Design review of the part built by this model. Coordinates are the model's own, in mm. A direction names the side the tool comes from. Coordinates: 2 decimals unless noted, no trailing zeros. Write each loop counter-clockwise with the first axis right and the second up, starting at its lowest first coordinate (ties: lowest second). Pieces come first, ordered by that corner, then holes. Notation, with made-up numbers: (66.25, -12.75) - (91.25, -12.75) arc R17 ccw to (91.25, -1.75) - close; hole circle Ø11 at (-34, 80.25). An arc over 180 degrees is marked (long way). Use a Markdown table: item, result.
from build123d import *

# Parameters (mm, degrees)
ESBO_O1_W                 = 50
ESBO_O1_H                 = 11
RESSALTO_EXTRUS_O1_DEPTH  = 22.5
ESBO_O2_W                 = 46
ESBO_O2_H                 = 7
CORTE_EXTRUS_O1_DEPTH     = 20.5
ESBO_O3_W                 = 10.97916057
ESBO_O3_H                 = 2
CORTE_EXTRUS_O2_DEPTH     = 4
CORTE_EXTRUS_O3_DEPTH     = 4
ESBO_O9_W                 = 50
ESBO_O9_H                 = 4
RESSALTO_EXTRUS_O4_DEPTH  = 7
ESBO_O13_R                = 1.5
CORTE_EXTRUS_O4_DEPTH     = 7
ESBO_O19_W                = 9
ESBO_O19_H                = 4
RESSALTO_EXTRUS_O5_DEPTH  = 22.5
ESBO_O20_W                = 50
ESBO_O20_H                = 4
CORTE_EXTRUS_O5_DEPTH     = 7
RESSALTO_EXTRUS_O6_DEPTH  = 0.75
RESSALTO_EXTRUS_O7_DEPTH  = 1.2
RESSALTO_EXTRUS_O8_DEPTH  = 1.5
RESSALTO_EXTRUS_O9_DEPTH  = 4.5
ESBO_O26_R                = 2.9
CORTE_EXTRUS_O6_DEPTH     = 4
ESBO_O28_W                = 7
ESBO_O28_H                = 7
RESSALTO_EXTRUS_O10_DEPTH = 4.5
CHANFRO1_SIZE             = 5
CHANFRO1_SIZE_2           = 3.372542584
CHANFRO2_SIZE             = 3.372542584
CHANFRO2_SIZE_2           = 5
CHANFRO3_SIZE             = 5
CHANFRO3_SIZE2            = 0.881634904
CHANFRO4_SIZE             = 5
CHANFRO4_SIZE2            = 1.919320175


with BuildPart() as part:
    # Esboço1 → Ressalto-extrusão1 (new body)
    with BuildSketch(Plane(origin=(0, 0, 0), x_dir=(1, 0, 0), z_dir=(0, 1, 0))):
        Rectangle(ESBO_O1_W, ESBO_O1_H)
    extrude(amount=RESSALTO_EXTRUS_O1_DEPTH)

    # Esboço2 → Corte-extrusão1 (cut)
    with BuildSketch(Plane(origin=(0, 22.5, 0), x_dir=(1, 0, 0), z_dir=(0, 1, 0))):
        Rectangle(ESBO_O2_W, ESBO_O2_H)
    extrude(amount=-CORTE_EXTRUS_O1_DEPTH, mode=Mode.SUBTRACT)

    # Esboço3 → Corte-extrusão2 (cut)
    with BuildSketch(Plane(origin=(0, 22.5, 0), x_dir=(1, 0, 0), z_dir=(0, 1, 0))):
        with Locations((0, 4.5)):
            Rectangle(ESBO_O3_W, ESBO_O3_H)
    extrude(amount=-CORTE_EXTRUS_O2_DEPTH, mode=Mode.SUBTRACT)

    # Esboço5 → Corte-extrusão3 (cut)
    with BuildSketch(Plane.XY.offset(5.5)):
        with BuildLine():
            Line((-21, 22.5), (-4.5, 22.5))
            Line((-4.5, 22.5), (-4.5, 11.75))
            ThreePointArc((-4.5, 11.75), (-12.75, 3.5), (-21, 11.75))
            Line((-21, 11.75), (-21, 22.5))
        make_face()
        with BuildLine():
            Line((4.5, 22.5), (21, 22.5))
            Line((21, 22.5), (21, 11.75))
            ThreePointArc((21, 11.75), (12.75, 3.5), (4.5, 11.75))
            Line((4.5, 11.75), (4.5, 22.5))
        make_face()
    extrude(amount=-CORTE_EXTRUS_O3_DEPTH, mode=Mode.SUBTRACT)

    # Esboço9 → Ressalto-extrusão4 (add)
    with BuildSketch(Plane(origin=(0, 0, -5.5), x_dir=(-1, 0, 0), z_dir=(0, 0, -1))):
        with Locations((0, 2)):
            Rectangle(ESBO_O9_W, ESBO_O9_H)
    extrude(amount=RESSALTO_EXTRUS_O4_DEPTH)

    # Esboço13 → Corte-extrusão4 (cut)
    with BuildSketch(Plane(origin=(0, 4, 0), x_dir=(1, 0, 0), z_dir=(0, 1, 0))):
        with Locations(Location((10, 9, 0), (0, 0, 270))):
            Circle(ESBO_O13_R)
        with Locations(Location((5, 9, 0), (0, 0, 270))):
            Circle(ESBO_O13_R)
        with Locations(Location((20, 9, 0), (0, 0, 270))):
            Circle(ESBO_O13_R)
        with Locations(Location((15, 9, 0), (0, 0, 270))):
            Circle(ESBO_O13_R)
        with Locations(Location((0, 9, 0), (0, 0, 270))):
            Circle(ESBO_O13_R)
        with Locations(Location((-5, 9, 0), (0, 0, 270))):
            Circle(ESBO_O13_R)
        with Locations(Location((-10, 9, 0), (0, 0, 270))):
            Circle(ESBO_O13_R)
        with Locations(Location((-15, 9, 0), (0, 0, 270))):
            Circle(ESBO_O13_R)
        with Locations(Location((-20, 9, 0), (0, 0, 270))):
            Circle(ESBO_O13_R)
    extrude(amount=-CORTE_EXTRUS_O4_DEPTH, mode=Mode.SUBTRACT)

    # Esboço19 → Ressalto-extrusão5 (add)
    with BuildSketch(Plane(origin=(0, 22.5, 0), x_dir=(1, 0, 0), z_dir=(0, 1, 0))):
        with Locations((0, -5.5)):
            Rectangle(ESBO_O19_W, ESBO_O19_H)
    extrude(amount=-RESSALTO_EXTRUS_O5_DEPTH)

    # Esboço20 → Corte-extrusão5 (cut)
    with BuildSketch(Plane(origin=(0, 0, -12.5), x_dir=(-1, 0, 0), z_dir=(0, 0, -1))):
        with Locations((0, 2)):
            Rectangle(ESBO_O20_W, ESBO_O20_H)
    extrude(amount=-CORTE_EXTRUS_O5_DEPTH, mode=Mode.SUBTRACT)

    # Esboço21 → Ressalto-extrusão6 (add)
    with BuildSketch(Plane(origin=(0, 22.5, 0), x_dir=(1, 0, 0), z_dir=(0, 1, 0))):
        Polygon((-21, -5.5), (-21, -3.5), (-23, -3.5), (-23, 3.5), (-5.489580285, 3.5), (-5.489580285, 5.5), (-25, 5.5), (-25, -5.5), align=None)
        Polygon((21, -3.5), (21, -5.5), (25, -5.5), (25, 5.5), (5.489580285, 5.5), (5.489580285, 3.5), (23, 3.5), (23, -3.5), align=None)
    extrude(amount=RESSALTO_EXTRUS_O6_DEPTH)

    # Esboço22 → Ressalto-extrusão7 (add)
    with BuildSketch(Plane(origin=(0, 23.25, 0), x_dir=(1, 0, 0), z_dir=(0, 1, 0))):
        Polygon((-24, 3.5), (-24, -5.5), (-25, -5.5), (-25, 5.5), (-5.489580285, 5.5), (-5.489580285, 4.5), (-23, 4.5), (-24, 4.5), align=None)
        Polygon((23, 4.5), (5.489580285, 4.5), (5.489580285, 5.5), (25, 5.5), (25, -5.5), (24, -5.5), (24, 3.5), (24, 4.5), align=None)
    extrude(amount=RESSALTO_EXTRUS_O7_DEPTH)

    # Esboço23 → Ressalto-extrusão8 (add)
    with BuildSketch(Plane(origin=(0, 24.45, 0), x_dir=(1, 0, 0), z_dir=(0, 1, 0))):
        Polygon((-24, 4.5), (-24, -5.5), (-25, -5.5), (-25, 5.5), (-5.489580285, 5.5), (-5.489580285, 4.5), align=None)
        Polygon((-23, 3.5), (-5.489580285, 3.5), (-5.489580285, 4.5), (-24, 4.5), (-24, -5.5), (-21, -5.5), (-21, -3.5), (-23, -3.5), align=None)
        Polygon((5.489580285, 5.5), (5.489580285, 4.5), (24, 4.5), (24, -5.5), (25, -5.5), (25, 5.5), align=None)
        Polygon((23, -3.5), (21, -3.5), (21, -5.5), (24, -5.5), (24, 4.5), (5.489580285, 4.5), (5.489580285, 3.5), (23, 3.5), align=None)
    extrude(amount=RESSALTO_EXTRUS_O8_DEPTH)

    # Esboço24 → Ressalto-extrusão9 (add)
    with BuildSketch(Plane.XZ):
        Polygon((0, 3.5), (-3.5, 3.5), (-3.5, 0), (-3.5, -3.5), (3.5, -3.5), (3.5, 3.5), align=None)
    extrude(amount=RESSALTO_EXTRUS_O9_DEPTH)

    # Esboço26 → Corte-extrusão6 (cut)
    with BuildSketch(Plane.XZ.offset(4.5)):
        with Locations(Location((0, 0, 0), (0, 0, 270))):
            Circle(ESBO_O26_R)
    extrude(amount=-CORTE_EXTRUS_O6_DEPTH, mode=Mode.SUBTRACT)

    # Esboço28 → Ressalto-extrusão10 (add)
    with BuildSketch(Plane.XZ):
        Polygon((-4.5, 5.5), (-9.5, 5.5), (-9.5, -5.5), (9.5, -5.5), (9.5, 5.5), (4.5, 5.5), (4.5, 7.5), (-4.5, 7.5), align=None)
        Rectangle(ESBO_O28_W, ESBO_O28_H, mode=Mode.SUBTRACT)
    extrude(amount=RESSALTO_EXTRUS_O10_DEPTH)

    # Chanfro1
    # the kernel refuses this chamfer: 5, 3.372542584 mm, written as the material it adds along each edge
    # the kernel refuses this chamfer: 5, 3.372542584 mm, written as the material it takes off along each edge
    with BuildSketch(Plane(origin=(-9.5, -4.5, 18.417545032), x_dir=(-0.021644705014774095, 0.9997657259302418, 0), z_dir=(0, 0, -1))) as chanfro1_2_piece_1_section:
        Polygon((CHANFRO1_SIZE * 0.99976572593, CHANFRO1_SIZE * 0.0216447050148), (-CHANFRO1_SIZE_2 * 0.0216447050161, CHANFRO1_SIZE_2 * 0.999765725993), (0, 0), align=None)
    chanfro1_2_piece_1 = extrude(amount=36.835090064, mode=Mode.PRIVATE)
    chanfro1_2_piece_1 = split(chanfro1_2_piece_1, bisect_by=Plane(origin=(-8.365599313, 0, 0), z_dir=(0, -1, 0)), keep=Keep.TOP, mode=Mode.PRIVATE)
    add(chanfro1_2_piece_1, mode=Mode.SUBTRACT)

    # Chanfro2
    # the kernel refuses this chamfer: 5, 3.372542584 mm, written as the material it takes off along each edge
    with BuildSketch(Plane(origin=(9.5, -4.5, -18.417545032), x_dir=(-0.9988697089125116, -0.04753214298802805, 0), z_dir=(0, 0, 1))) as chanfro2_piece_1_section:
        Polygon((CHANFRO2_SIZE * 0.998869708975, -CHANFRO2_SIZE * 0.047532142991), (-CHANFRO2_SIZE_2 * 0.047532142988, -CHANFRO2_SIZE_2 * 0.998869708913), (0, 0), align=None)
    chanfro2_piece_1 = extrude(amount=36.835090064, mode=Mode.PRIVATE)
    chanfro2_piece_1 = split(chanfro2_piece_1, bisect_by=Plane(origin=(8.383687283, 0, 0), z_dir=(0, -1, 0)), keep=Keep.TOP, mode=Mode.PRIVATE)
    add(chanfro2_piece_1, mode=Mode.SUBTRACT)

    # Chanfro3
    chanfro3_edges = [part.edges().sort_by_distance(p)[0] for p in [
        (0, -4.5, -5.5),
    ]]
    chanfro3_side = [part.faces().sort_by_distance(p)[0] for p in [
        (0, 11.578416309, -5.5),
    ]]
    chamfer(chanfro3_edges, length=CHANFRO3_SIZE, length2=CHANFRO3_SIZE2, reference=chanfro3_side[0])

    # Chanfro4
    chanfro4_edges = [part.edges().sort_by_distance(p)[0] for p in [
        (0, -4.5, 7.5),
    ]]
    chanfro4_side = [part.faces().sort_by_distance(p)[0] for p in [
        (0, 9, 7.5),
    ]]
    chamfer(chanfro4_edges, length=CHANFRO4_SIZE, length2=CHANFRO4_SIZE2, reference=chanfro4_side[0])


solid = part.part
(1) For pin 1 (1 mm diameter, centred on x = 6, z = 3.5, fed in from +Y); pin 2 (10 mm diameter, centred on x = -15, y = 7.5, fed in from +Z); pin 3 (1.2 mm diameter, centred on x = 0, z = 5, fed in from +Y), all flat-tipped, find the tip position at first contact; note any pin that passes through.
Determined:
| item | result |
|---|---|
| pin 1 | y = 7.81 |
| pin 2 | z = 5.5 |
| pin 3 | y = 22.5 |
(2) For L1, parallel to X at y = 15.5, z = -1; L2, parallel to Z at x = 2, y = 14.5; L3, parallel to Y at x = -21.5, z = 5.25, list the stretches that pass through material, from the lowest coordinate up. Write a range as from..to.
Determined:
| item | result |
|---|---|
| L1 | -25..-23, 23..25 |
| L2 | -5.5..-3.5, 3.5..7.5 |
| L3 | 0..23.25, 24.45..25.95 |
(3) Take a section at C-C on y = 19. Write out the cut boundary in (x, z).
Determined:
| item | result |
|---|---|
| outline | (-25, -5.5) - (-5.49, -5.5) - (-5.49, -3.5) - (-23, -3.5) - (-23, 3.5) - (-21, 3.5) - (-21, 5.5) - (-25, 5.5) - close; (-4.5, 3.5) - (4.5, 3.5) - (4.5, 7.5) - (-4.5, 7.5) - close; (5.49, -5.5) - (25, -5.5) - (25, 5.5) - (21, 5.5) - (21, 3.5) - (23, 3.5) - (23, -3.5) - (5.49, -3.5) - close |
(4) Take a section at B-B on x = -12.75. Write out the cut boundary in (y, z), and give its area (3 significant figures).
Determined:
| item | result |
|---|---|
| outline | (0, -5.41) - (0.5, -5.5) - (25.95, -5.5) - (25.95, -3.5) - (24.45, -3.5) - (24.45, -4.5) - (23.25, -4.5) - (23.25, -3.5) - (2, -3.5) - (2, 3.5) - (3.5, 3.5) - (3.5, 5.5) - (0, 5.5) - close |
| area | 71.7 mm2 |
(5) Take a section at D-D on z = 1.25. Write out the cut boundary in (x, y), and give its area (3 significant figures).
Determined:
| item | result |
|---|---|
| outline | (-25, 0) - (-9.16, 0) - (-6.13, -4.5) - (-2.62, -4.5) - (-2.62, -0.5) - (2.62, -0.5) - (2.62, -4.5) - (6.13, -4.5) - (9.16, 0) - (25, 0) - (25, 25.95) - (23, 25.95) - (23, 24.45) - (24, 24.45) - (24, 23.25) - (23, 23.25) - (23, 2) - (-23, 2) - (-23, 23.25) - (-24, 23.25) - (-24, 24.45) - (-23, 24.45) - (-23, 25.95) - (-25, 25.95) - close |
| area | 241 mm2 |
(6) Draft analysis for pull direction X (two halves, no side actions). For faces 6 (the flat face through (0, 12, -3.5)), 7 (the flat face through (23, 25, 0)), 8 (the flat face through (-0.35, -1.48, -5.15)), state which applies: +X half, -X half, draft (parallel to the pull), parting line (faces both ways), or undercut.
Determined:
| item | result |
|---|---|
| face 6 | undercut |
| face 7 | undercut |
| face 8 | draft |
(7) Machinability: for faces 1 (the flat face through (5.49, 22, -4)), 2 (the cylindrical face through (0.1, -2.5, 2.9)), 3 (the flat face through (17, 23.25, -4)), 4 (the flat face through (-23, 12, 0)), 5 (the flat face through (21, 18, 5)), which of the approach directions +Z, -Z, +X, -X, +Y, -Y give a long, thin tool a straight path to every point of the face, cutting with its end or side? Answer none if there is none.
Determined:
| item | result |
|---|---|
| face 1 | +Z, -Z, +Y |
| face 2 | -Y |
| face 3 | +Z |
| face 4 | +Y |
| face 5 | +Z, +Y |
(8) Take a section at A-A on y = 13. Write out the cut boundary in (x, z).
Determined:
| item | result |
|---|---|
| outline | (-25, -5.5) - (25, -5.5) - (25, 5.5) - (21, 5.5) - (21, 3.5) - (23, 3.5) - (23, -3.5) - (-23, -3.5) - (-23, 3.5) - (-21, 3.5) - (-21, 5.5) - (-25, 5.5) - close; (-4.5, 3.5) - (4.5, 3.5) - (4.5, 7.5) - (-4.5, 7.5) - close |
